Geometry check sheet. Reference: the model listing, model coordinates, mm. Face numbers are marked on the shaded views. Round coordinates to 2 decimals unless told otherwise and drop trailing zeros. Order: outer loops, then holes, each group sorted by start corner. A loop starts at its lowest first (then second) coordinate and runs counter-clockwise, first axis right, second up. Notation, with made-up numbers: (89.5, -7) - (103.5, -7) arc R14 ccw to (103.5, 0) - close; hole circle Ø8 at (88.25, 21). An arc over 180 degrees is marked (long way). Return JSON: item names as keys, results as strings. Group by question number.
Q1. Sectioned sample at D-D, the plane x = -16.5. Record the cut outline in (y, z).
Q2. Sectioned sample at A-A, the plane x = 0. Record the cut outline in (y, z), then the cut area to 3 significant figures.
Q3. Draft check along X on the marked faces 1, 2 and 3. Enter one of: pulls with the +X half, pulls with the -X half, needs draft (parallel to the pull), parting line crosses it, or undercut.
Q4. Material ranges on line 1 along X through (y, z) = (-6.5, -45); line 2 along Z through (x, y) = (0, 2); line 3 along X through (y, z) = (2.25, 52), recorded low to high.
Q5. Gauge pin test, flat end, axial feed: pin 1 Ø12 at (x, y) = (9, 9) entering from +Z. Record the tip position at first contact, or that the pin passes through.
Q6. Sectioned sample at C-C, the plane z = -45. Record the cut outline in (x, y), then the cut area to 4 significant figures.
Q7. Sectioned sample at B-B, the plane y = 7.5. Record the cut outline in (x, z), then the cut area to 3 significant figures.
Autodesk Inventor part; units mm, degrees
ref_plane "YZ Plane" through (0, 0, 0) normal (1, 0, 0) x (0, 1, 0)
ref_plane "XZ Plane" through (0, 0, 0) normal (0, 1, 0) x (-1, 0, 0)
ref_plane "XY Plane" through (0, 0, 0) normal (0, 0, 1) x (1, 0, 0)
sketch "Sketch1" plane through (0, 0, 0) normal (0, 1, 0) x (-1, 0, 0)
  line L0 (30, -50) -> (-30, -50)
  line L1 (-30, -50) -> (-30, 50)
  arc A0 (30, 50) -> (-30, 50) centre (0, 50) ccw
  line L2 (30, 50) -> (30, -50)
  circle A1 centre (0, 50) radius 15
  point P0 (0, 0)
  point P1 (30, 0)
  dimension "d0" = 60
  dimension "d1" = 100
  dimension "d2" = 30
extrude "Extrusion1" add sketch "Sketch1" along normal mid plane 25
sketch "Sketch2" plane through (0, 0, 0) normal (0, 1, 0) x (-1, 0, 0)
  line L0 (-30, -50) -> (-30, 50) construction
  arc A0 (30, 50) -> (-30, 50) centre (0, 50) ccw construction
  line L1 (30, 50) -> (30, -50) construction
  line L2 (30, -50) -> (-30, -50) construction
  circle A1 centre (0, 50) radius 15 construction
  line L3 (30, 50) -> (30, -50) construction
  line L4 (30, -40) -> (-30, -40) construction
  line L5 (-30, -50) -> (-30, 50) construction
  line L6 (0, -40) -> (0, -50) construction
  circle A2 centre (15, -45) radius 4.05
  circle A3 centre (-15, -45) radius 4.05
  point P0 (0, 0)
  point P1 (0, -45)
  dimension "d5" = 10
  dimension "d6" = 8.1
  dimension "d7" = 30
extrude "Extrusion2" cut sketch "Sketch2" along normal through all both and the other way through all
properties part number "element2_obj4"
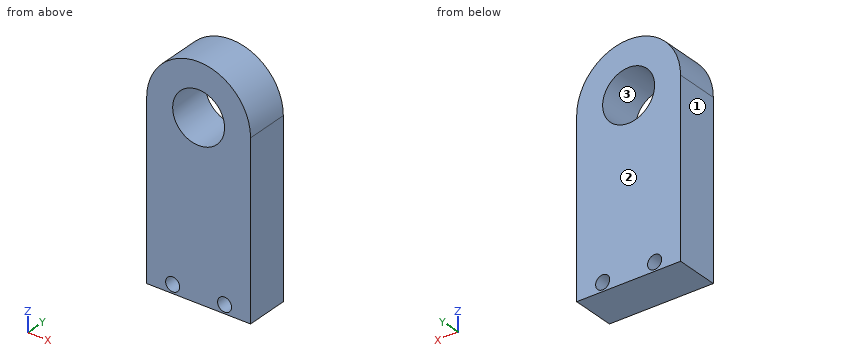
Reply:
{
 "1": {"outline": "(-12.5, -50) - (12.5, -50) - (12.5, -48.76) - (-12.5, -48.76) - close; (-12.5, -41.24) - (12.5, -41.24) - (12.5, 75.05) - (-12.5, 75.05) - close"},
 "2": {"outline": "(-12.5, -50) - (12.5, -50) - (12.5, 35) - (-12.5, 35) - close; (-12.5, 65) - (12.5, 65) - (12.5, 80) - (-12.5, 80) - close", "area": "2,500 mm^2"},
 "3": {"face 1": "pulls with the -X half", "face 2": "needs draft", "face 3": "undercut"},
 "4": {"line 1": "-30 to -19.05, -10.95 to 10.95, 19.05 to 30", "line 2": "-50 to 35, 65 to 80", "line 3": "-29.93 to -14.87, 14.87 to 29.93"},
 "5": {"pin 1": "z = 79.85"},
 "6": {"outline": "(-30, -12.5) - (-19.05, -12.5) - (-19.05, 12.5) - (-30, 12.5) - close; (-10.95, -12.5) - (10.95, -12.5) - (10.95, 12.5) - (-10.95, 12.5) - close; (19.05, -12.5) - (30, -12.5) - (30, 12.5) - (19.05, 12.5) - close", "area": "1,095 mm^2"},
 "7": {"outline": "(-30, -50) - (30, -50) - (30, 50) arc R30 ccw to (-30, 50) - close; hole circle Ø8.1 at (-15, -45); hole circle Ø30 at (0, 50); hole circle Ø8.1 at (15, -45)", "area": "6,600 mm^2"}
}
